Autodesk Inventor part; units mm, degrees
ref_plane "IDS_WORKPLANE{1}" through (0, 12.7, 0) normal (0, 1, 0) x (-1, 0, 0)
ref_plane "IDS_WORKPLANE{2}" through (5.5563, 0, 0) normal (-1, 0, 0) x (0, 0, 1)
ref_plane "YZ Plane" through (0, 0, 0) normal (1, 0, 0) x (0, 1, 0)
sketch "Boceto1" plane through (0, 0, 0) normal (0, 0, 1) x (1, 0, 0)
  line L0 (0, 12.7) -> (11.1125, 12.7)
  line L1 (-1.9497, 0) -> (21.5466, 0)
  line L2 (0, 12.7) -> (0, 6.35)
  line L3 (0, 6.35) -> (11.1125, 6.35)
  line L4 (11.1125, 6.35) -> (11.1125, 12.7)
  line L5 (-6.6489, 0) -> (26.2458, 0)
  line L6 (0, 54) -> (0, -9)
  dimension "d0" = 25.4
  dimension "d1" = 12.7
  dimension "d2" = 11.1125
revolve "Cuerpo" add sketch "Boceto1" angle 360 about axis through (-1.9497, 0, 0) along (1, 0, 0)
ref_plane "IDS_WORKPLANE{1}" through (0, 12.7, 0) normal (0, 1, 0) x (-1, 0, 0)
sketch "Boceto2" plane through (0, 12.7, 0) normal (0, 1, 0) x (-1, 0, 0)
  line L0 (0, 12.7) -> (0, -12.7)
  line L1 (-12.156, 0) -> (2.026, 0)
  point P0 (-5.5563, 0)
  dimension "d7" = 5.5563
hole "Agujero1" at (5.5563, 12.7, 0) direction (0, -1, 0) diameter 6.35 depth 12.7 tip angle 118
ref_plane "IDS_WORKPLANE{2}" through (5.5563, 0, 0) normal (-1, 0, 0) x (0, 0, 1)
sketch "Boceto3" plane through (5.5563, 0, 0) normal (-1, 0, 0) x (0, 0, 1)
  line L0 (0, 12.7) -> (1.7831, 12.7)
  line L1 (1.7831, 12.7) -> (3.175, 12.4041)
  line L2 (3.175, 12.4041) -> (3.175, 7.1157)
  line L3 (0, 56.54) -> (0, -24.24)
  circle A0 centre (0, 0) radius 12.7
  line L4 (0, 12.7) -> (0, 6.35)
  line L5 (3.175, 7.1157) -> (0.3175, 6.35)
  line L6 (0.3175, 6.35) -> (0, 6.35)
  dimension "d18" = 3.5662
  dimension "d19" = 6.35
  dimension "d20" = 0.635
  dimension "d21" = 6.35
  dimension "d30" = 15
  dimension "d31" = 12
revolve "Tornillo de cabeza perdida1" add sketch "Boceto3" angle 360 about axis through (5.5563, 12.7, 0) along (0, -1, 0) picked at (1.5203, 8.7069) contours A0 L2 L5 L6 L3 | L0 L1 L2 A0
sketch "Boceto4" plane through (0, 12.7, 0) normal (0, 1, 0) x (-1, 0, 0)
  line L0 (-5.5562, 1.27) -> (-4.4564, 0.635)
  line L1 (-4.4564, 0.635) -> (-4.4564, -0.635)
  line L2 (-4.4564, -0.635) -> (-5.5563, -1.27)
  line L3 (-5.5563, -1.27) -> (-6.6561, -0.635)
  line L4 (-6.6561, -0.635) -> (-6.6561, 0.635)
  line L5 (-6.6561, 0.635) -> (-5.5562, 1.27)
  line L6 (-14.2345, 0) -> (2.3724, 0)
  line L7 (0, 6.35) -> (0, -6.35)
  point P0 (-5.5563, 0)
  dimension "d22" = 2.54
  dimension "d23" = 5.5563
extrude "Ranura1" cut sketch "Boceto4" against normal blind 1.5875
chamfer "Chaflán1" distance 1.1112 angle 15 1 edges at (11.1125, -12.7, 0) measured on face at (3.7042, 10.7339, 6.7877)
chamfer "Chaflán2" distance 0.1905 distance2 1.1112 1 edges at (11.1125, -6.35, 0) measured on face at (11.1125, 10.2032, -1.4959)
fillet "Empalme1" radius 0.5558 1 edges at (0, -12.7, 0)
equation "\"d18\" = GD1"
equation "\"d19\" = NND"
equation "\"d20\" = 0.1 * NND"
equation "\"d21\" = -0.5 * WND + 0.5 * SD2"
equation "\"d30\" = FAWI"
equation "\"d31\" = 0.8 * FAWI"
equation "\"d22\" = 0.4 * NND"
equation "\"d24\" = 0.25 * NND"
equation "\"d8\" = NND"
equation "\"d13\" = 0.5 * SD2"
equation "\"d4\" = PHH"
equation "\"d5\" = FAWI"
equation "\"d59\" = PHH"
equation "\"d26\" = -0.5 * WND + 0.5 * NND1"
equation "\"d27\" = PHH"
equation "\"d29\" = RR"
equation "\"d0\" = SD2"
equation "\"d1\" = WND"
equation "\"d2\" = SD"
equation "\"WND\" = 12.7"
equation "\"SD2\" = 25.4"
equation "\"SD\" = 11.1125"
equation "\"NND\" = 6.35"
equation "\"FAWI\" = 15deg"
equation "\"PHH\" = 1.11125"
equation "\"d6\" = 0.5 * SD2"
equation "\"GD1\" = 3.56616"
equation "\"d17\" = -0.5 * SD"
equation "\"RR\" = 0.55575"
equation "\"NND1\" = 13.081"
properties part number "Unbrako. Hallowell Steel Collars. Inch Series - 0.5 x 1 x 7/16" material "Acero, suave"
Read the model definition and answer for the solid it produces. Units are mm, in the model's axes. A direction names the side the tool comes from. Give positions to 0.01 mm unless a question says otherwise; leave off trailing zeros. Write each loop counter-clockwise with the first axis right and the second up, starting at its lowest first coordinate (ties: lowest second). Pieces come first, ordered by that corner, then holes. Notation, with made-up numbers: (16, -28) - (38, -28) arc R20 ccw to (38, 11) - close; hole circle Ø2 at (45, 0.5). An arc over 180 degrees is marked (long way). Answer in a Markdown table with one row per item. Add a question column.
Item 1: Section C-C, the plane x = 1.5 is taken. Write down the section's boundary in (y, z), and give its area (3 significant figures).
Item 2: A tool of negligible diameter and unlimited length cuts with its end or side. For faces 1 (the face through (11.112, 5, -5)), 2 (the face through (6.099, 11.917, -0.957)), from which of +Z, -Z, +X, -X, +Y, -Y can it reach the whole face along a straight path? Write none if from no direction.
Item 3: Flat-ended cylindrical pins translate along their axes: P1, Ø1.1, axis at x = 5.5, z = 0.5, coming from the +Y side; P2, Ø2, axis at x = 3, y = 2.5, coming from the -Z side; P3, Ø11.5, axis at y = 0, z = 0, coming from the +X side; P4, Ø6, axis at x = 3, y = -6, coming from the +Z side. Find the tip coordinate at first contact, or state that the pin passes through.
Item 4: Determine the mould class of faces 3 (the face through (5.1, 6.4, 0.2)), 4 (the face through (7, 12.7, 0)), 5 (the face through (0, 5, -5)) for opening direction Y: pulls with the +Y half, pulls with the -Y half, needs draft (parallel to the pull), parting line crosses it, or undercut.
Item 5: Section A-A, the plane y = 0 is taken. Write down the section's boundary in (x, z).
Item 6: Find the intervals of material crossed by L1, parallel to Z at x = 3.25, y = 0; L2, parallel to Z at x = 3, y = 3.25; L3, parallel to Y at x = 1, z = -3, in increasing order.
Recorded:
| question | item | result |
|---|---|---|
| 1 | outline | circle Ø25.4 at (0, 0); hole circle Ø12.7 at (0, 0) |
| 1 | area | 380 mm2 |
| 2 | face 1 | +Z, -Z, +X, +Y, -Y |
| 2 | face 2 | +Y |
| 3 | P1 | stops at y = 11.11 |
| 3 | P2 | stops at z = -12.61 |
| 3 | P3 | passes through |
| 3 | P4 | stops at z = 12.34 |
| 4 | face 3 | undercut |
| 4 | face 4 | pulls with the +Y half |
| 4 | face 5 | needs draft |
| 5 | outline | (0, -12.14) arc R0.56 ccw to (0.56, -12.7) - (10, -12.7) - (11.11, -12.4) - (11.11, -6.54) - (10, -6.35) - (0, -6.35) - close; (0, 6.35) - (10, 6.35) - (11.11, 6.54) - (11.11, 12.4) - (10, 12.7) - (0.56, 12.7) arc R0.56 ccw to (0, 12.14) - close |
| 6 | L1 | z = -12.7 to -6.35, 6.35 to 12.7 |
| 6 | L2 | z = -12.28 to -5.46, 5.46 to 12.28 |
| 6 | L3 | y = -12.34 to -5.6, 5.6 to 12.34 |
